Verification items for the finished model (mm, model axes). Round coordinates to 2 decimals unless told otherwise and drop trailing zeros. Write each loop counter-clockwise with the first axis right and the second up, starting at its lowest first coordinate (ties: lowest second). Pieces come first, ordered by that corner, then holes. Notation, with made-up numbers: (48, 5) - (62, 5) arc R22 ccw to (62, 35) - close; hole circle Ø11 at (16, 28.5). An arc over 180 degrees is marked (long way). Answer as a JSON object with one key per item and string values.
```python
from build123d import *

# Parameters (mm, degrees)
F1_DEPTH = 21
F2_R     = 3


with BuildPart() as f1:
    # F0 (on Front) → F1 (new body)
    with BuildSketch(Plane.XZ):
        with BuildLine():
            Line((400, 0), (381.3953488372, 80))
            Line((381.3953488372, 80), (89.5979005098, 80))
            ThreePointArc((89.5979005098, 80), (86.0623666039, 81.4644660941), (84.5979005098, 85))
            Line((84.5979005098, 85), (84.5979005098, 352.7062674352))
            ThreePointArc((84.5979005098, 352.7062674352), (88.7932713354, 364.9624371736), (99.6192701756, 372.0766892167))
            Line((99.6192701756, 372.0766892167), (214.9680088476, 401.7238871894))
            ThreePointArc((214.9680088476, 401.7238871894), (223.0875079778, 407.0595762217), (226.2340360969, 416.2517035256))
            Line((226.2340360969, 416.2517035256), (226.2340360969, 430))
            Line((226.2340360969, 430), (0, 430))
            Line((0, 430), (0, 0))
            Line((0, 0), (85, 0))
            Line((85, 0), (85, 35))
            ThreePointArc((85, 35), (86.4644660941, 38.5355339059), (90, 40))
            Line((90, 40), (337.2612395977, 40))
            ThreePointArc((337.2612395977, 40), (340.4311835928, 38.8667111436), (342.1641427058, 35.9805820273))
            Line((342.1641427058, 35.9805820273), (349.360269427, 0))
            Line((349.360269427, 0), (400, 0))
        make_face()
    extrude(amount=F1_DEPTH)

    # F2
    f2_edges = [f1.edges().sort_by_distance(p)[0] for p in [
        (226.234036, -21, 423.125852),
        (113.117018, -21, 430),
        (0, -21, 215),
        (42.5, -21, 0),
        (85, -21, 17.5),
        (86.464466, -21, 38.535534),
        (213.63062, -21, 40),
        (340.431184, -21, 38.866711),
        (345.762206, -21, 17.990291),
        (374.680135, -21, 0),
        (390.697674, -21, 40),
        (235.496625, -21, 80),
        (86.062367, -21, 81.464466),
        (84.597901, -21, 218.853134),
        (88.793271, -21, 364.962437),
        (157.29364, -21, 386.900288),
        (223.087508, -21, 407.059576),
        (226.234036, 0, 423.125852),
        (113.117018, 0, 430),
        (0, 0, 215),
        (42.5, 0, 0),
        (85, 0, 17.5),
        (86.464466, 0, 38.535534),
        (213.63062, 0, 40),
        (340.431184, 0, 38.866711),
        (345.762206, 0, 17.990291),
        (374.680135, 0, 0),
        (390.697674, 0, 40),
        (235.496625, 0, 80),
        (86.062367, 0, 81.464466),
        (84.597901, 0, 218.853134),
        (88.793271, 0, 364.962437),
        (157.29364, 0, 386.900288),
        (223.087508, 0, 407.059576),
    ]]
    fillet(f2_edges, radius=F2_R)


solid = f1.part
```
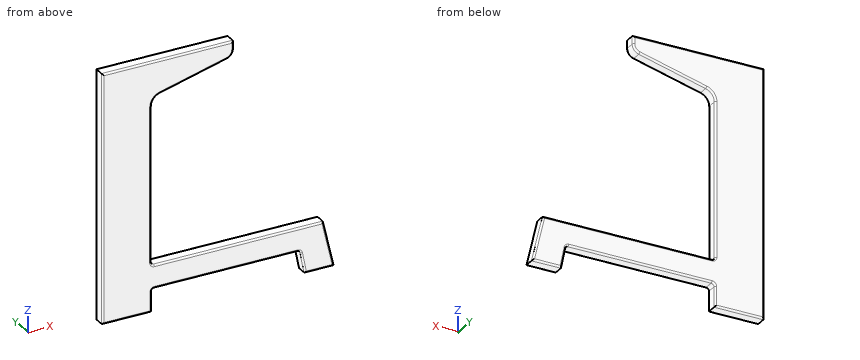
Q1. Gauge pin test, flat ends, axial feed: P1, Ø12, axis at x = 237, y = -16.5, coming from the -Z side; P2, Ø12, axis at y = -10, z = 150.5, coming from the +X side. Record the tip position at first contact, or that the pin passes through.
Geometry check:
{"P1": "stops at z = 40", "P2": "stops at x = 84.6"}
Q2. Section check C-C, the plane y = -9.5. Record the cut outline in (x, z).
Geometry check:
{"outline": "(0, 0) - (85, 0) - (85, 35) arc R5 cw to (90, 40) - (337.26, 40) arc R5 cw to (342.16, 35.98) - (349.36, 0) - (400, 0) - (381.4, 80) - (89.6, 80) arc R5 cw to (84.6, 85) - (84.6, 352.71) arc R20 cw to (99.62, 372.08) - (214.97, 401.72) arc R15 ccw to (226.23, 416.25) - (226.23, 430) - (0, 430) - close"}
Q3. Section check B-B, the plane z = 168. Record the cut outline in (x, y), then the cut area to 3 significant figures.
Geometry check:
{"outline": "(0, -18) arc R3 ccw to (3, -21) - (81.6, -21) arc R3 ccw to (84.6, -18) - (84.6, -3) arc R3 ccw to (81.6, 0) - (3, 0) arc R3 ccw to (0, -3) - close", "area": "1,770 mm2"}
Q4. Material ranges on line 1 along X through (y, z) = (-8.75, 233); line 2 along Z through (x, y) = (357, -5.25); line 3 along Z through (x, y) = (145, -15.75), recorded low to high. Write a range as [from, to].
Geometry check:
{"line 1": "x = [0, 84.6]", "line 2": "z = [0, 80]", "line 3": "z = [40, 80], [383.74, 430]"}
Q5. Section check A-A, the plane x = 308. Record the cut outline in (y, z), then the cut area to 3 significant figures.
Geometry check:
{"outline": "(-21, 43) arc R3 ccw to (-18, 40) - (-3, 40) arc R3 ccw to (0, 43) - (0, 77) arc R3 ccw to (-3, 80) - (-18, 80) arc R3 ccw to (-21, 77) - close", "area": "832 mm2"}
